from build123d import *

# Parameters (mm, degrees)
BOX003_W        = 52
BOX003_H        = 38
BOX003_DEPTH    = 16.1
SKETCH018_R     = 4.2
SKETCH018_W     = 19
SKETCH018_H     = 10
POCKET010_DEPTH = 38.001
SKETCH020_R     = 1.4
SKETCH020_R_2   = 1.68
POCKET011_DEPTH = 16.101
SKETCH021_R     = 1.5
POCKET012_DEPTH = 3
SKETCH019_R     = 1.5
POCKET013_DEPTH = 3
FILLET006_R     = 5


with BuildPart() as part:
    # Box003 → Box003 (new body)
    with BuildSketch(Plane(origin=(70, 0, 0), x_dir=(1, 0, 0), z_dir=(0, 0, 1))):
        with Locations((26, 19)):
            Rectangle(BOX003_W, BOX003_H)
    extrude(amount=BOX003_DEPTH)

    # Sketch018 → Pocket010 (cut, through all)
    with BuildSketch(Plane(origin=(70, 38, 0), x_dir=(-1, 0, 0), z_dir=(0, 1, 0))):
        with Locations((-46, 8.25)):
            Circle(SKETCH018_R)
        with Locations((-6, 8.25)):
            Circle(SKETCH018_R)
        with Locations((-26, 8.1)):
            Rectangle(SKETCH018_W, SKETCH018_H)
    extrude(amount=-POCKET010_DEPTH, mode=Mode.SUBTRACT)

    # Sketch020 → Pocket011 (cut, through all)
    with BuildSketch(Plane(origin=(70, 0, 16.1), x_dir=(1, 0, 0), z_dir=(0, 0, 1))):
        with Locations((13, 5)):
            Circle(SKETCH020_R)
        with Locations((39, 5)):
            Circle(SKETCH020_R)
        with Locations((39, 33)):
            Circle(SKETCH020_R)
        with Locations((13, 33)):
            Circle(SKETCH020_R)
        with Locations((26, 4)):
            Circle(SKETCH020_R_2)
        with Locations((26, 17.2)):
            Circle(SKETCH020_R_2)
    extrude(amount=-POCKET011_DEPTH, mode=Mode.SUBTRACT)

    # Sketch021 → Pocket012 (cut)
    with BuildSketch(Plane(origin=(70, 0, 0), x_dir=(0, -1, 0), z_dir=(-1, 0, 0))):
        with Locations((-29.5, 8.25)):
            Circle(SKETCH021_R)
        with Locations((-9.5, 8.25)):
            Circle(SKETCH021_R)
    extrude(amount=-POCKET012_DEPTH, mode=Mode.SUBTRACT)

    # Sketch019 → Pocket013 (cut)
    with BuildSketch(Plane.YZ.offset(122)):
        with Locations((9.5, 8.25)):
            Circle(SKETCH019_R)
        with Locations((29.5, 8.25)):
            Circle(SKETCH019_R)
    extrude(amount=-POCKET013_DEPTH, mode=Mode.SUBTRACT)

    # Fillet006
    fillet006_edges = [part.edges().sort_by_distance(p)[0] for p in [
        (122, 19, 16.1),
        (122, 19, 0),
        (70, 19, 0),
        (70, 19, 16.1),
    ]]
    fillet(fillet006_edges, radius=FILLET006_R)


solid = part.part
For this review, take the finished solid that the model builds, in its own axes (mm). A direction names the side the tool comes from. Round coordinates to 2 decimals unless told otherwise and drop trailing zeros. Order: outer loops, then holes, each group sorted by start corner. A loop starts at its lowest first (then second) coordinate and runs counter-clockwise, first axis right, second up. Notation, with made-up numbers: M -2,85 L 14,85 A21 ccw 14,113 Z; hole C -40,19.5 d4. An arc over 180 degrees is marked long. Write each question's results on one line, items separated by ' | '. Start each with the question number.
1. Add section A-A (y = 9.5). State the section outline as (x, z) points, then the cut area to 3 significant figures.
2. Clearance check with flat-ended pins moving along their axes: pin 1 Ø5 at (y, z) = (20, 14) entering from -X; pin 2 Ø2.5 at (y, z) = (29.5, 8.25) entering from +X. State where each tip first meets the part, or that it passes through.
3. To check wall thickness, follow L1, parallel to Y at x = 109, z = 3.75; L2, parallel to Y at x = 71.7, z = 8.25; L3, parallel to X at y = 34.5, z = 8.5. State the ranges of each line that lie inside material, in increasing order. Write a range as [from, to].
4. Add section D-D (x = 116). State the section outline as (y, z) points.
5. Draft analysis for pull direction Z (two halves, no side actions). For faces 1 (the face through (96.1, 19.3, 13.1)), 2 (the face through (95.7, 19.3, 16.1)), 3 (the face through (95.6, 0, 2.6)), state which applies: pulls with the +Z half, pulls with the -Z half, needs draft (parallel to the pull), parting line crosses it, or undercut.
6. Add section B-B (x = 96). State the section outline as (y, z) points.
7. Tool access review of faces 4 (the face through (120.5, 19.27, 14.67)), 5 (the face through (120.976, 10.886, 7.675)), 6 (the face through (86.5, 19, 8)), 7 (the face through (71.024, 28.114, 7.675)): name each direction out of +Z, -Z, +X, -X, +Y, -Y from which nothing blocks a thin tool from reaching the whole face with its end or side.
8. Add section C-C (x = 109). State the section outline as (y, z) points.
Output values:
1) outline: M 70,5 A5 ccw 75,0 L 117,0 A5 ccw 122,5 L 122,6.75 L 119.92,6.75 A4.2 cw long 119.92,9.75 L 122,9.75 L 122,11.1 A5 ccw 117,16.1 L 75,16.1 A5 ccw 70,11.1 L 70,9.75 L 72.08,9.75 A4.2 cw long 72.08,6.75 L 70,6.75 Z; hole M 86.5,3.1 L 105.5,3.1 L 105.5,13.1 L 86.5,13.1 Z | area: 504 mm^2
2) pin 1: x = 70.02 | pin 2: x = 111.99
3) L1: [0, 3.6], [6.4, 31.6], [34.4, 38] | L2: [0, 8], [11, 28], [31, 38] | L3: [70, 71.81], [80.19, 86.5], [105.5, 111.81], [120.19, 122]
4) outline: M 0,0 L 38,0 L 38,4.05 L 0,4.05 Z; M 0,12.45 L 38,12.45 L 38,16.1 L 0,16.1 Z
5) face 1: undercut | face 2: pulls with the +Z half | face 3: needs draft
6) outline: M 0,0 L 2.32,0 L 2.32,3.1 L 0,3.1 Z; M 0,13.1 L 2.32,13.1 L 2.32,16.1 L 0,16.1 Z; M 5.68,0 L 15.52,0 L 15.52,3.1 L 5.68,3.1 Z; M 5.68,13.1 L 15.52,13.1 L 15.52,16.1 L 5.68,16.1 Z; M 18.88,0 L 38,0 L 38,3.1 L 18.88,3.1 Z; M 18.88,13.1 L 38,13.1 L 38,16.1 L 18.88,16.1 Z
7) face 4: +Z, +X, +Y, -Y | face 5: +X | face 6: +Y, -Y | face 7: -X
8) outline: M 0,0 L 3.6,0 L 3.6,16.1 L 0,16.1 Z; M 6.4,0 L 31.6,0 L 31.6,16.1 L 6.4,16.1 Z; M 34.4,0 L 38,0 L 38,16.1 L 34.4,16.1 Z
